The figure shows three views and two pictorial views of one solid part (mm, origin at its lowest corner). Answer the questions. Coordinates: 2 decimals unless noted, no trailing zeros. Loops run counter-clockwise (first coordinate to the right, second up) from the corner with the lowest first, then second, coordinate; pieces in that order, holes last. Notation, with made-up numbers: M 19,35 L 64,35 A34 ccw 64,72 Z; hole C 78.5,32 d1. An arc over 180 degrees is marked long. Return JSON: item names as keys, results as strings. Group by question number.
1. Section D-D (x = 28.5) is taken. Write down the section's boundary in (y, z).
2. Straight lines are drawn through the part: L1, parallel to Z at x = 3, y = 8; L2, parallel to Z at x = 12, y = 2.5; L3, parallel to X at y = 3.5, z = 6.5. For each, find the intervals that lie inside material, in ascending order. Write a range as from..to.
3. Section A-A (z = 15) is taken. Write down the section's boundary in (x, y), then the cut area to 3 significant figures.
4. Section B-B (x = 15) is taken. Write down the section's boundary in (y, z).
5. Given P1, Ø3.5, axis at x = 27, z = 3, coming from the +Y side, flat-ended and moving along its own axis, determine where the tip first touches the part or whether it passes through.
6. Section C-C (y = 1.25) is taken. Write down the section's boundary in (x, z), then the cut area to 3 significant figures.
7. The mould has two halves that part along Z. Classify the marked faces 1, 2 and 3: pulls with the +Z half, pulls with the -Z half, needs draft (parallel to the pull), parting line crosses it, or undercut.
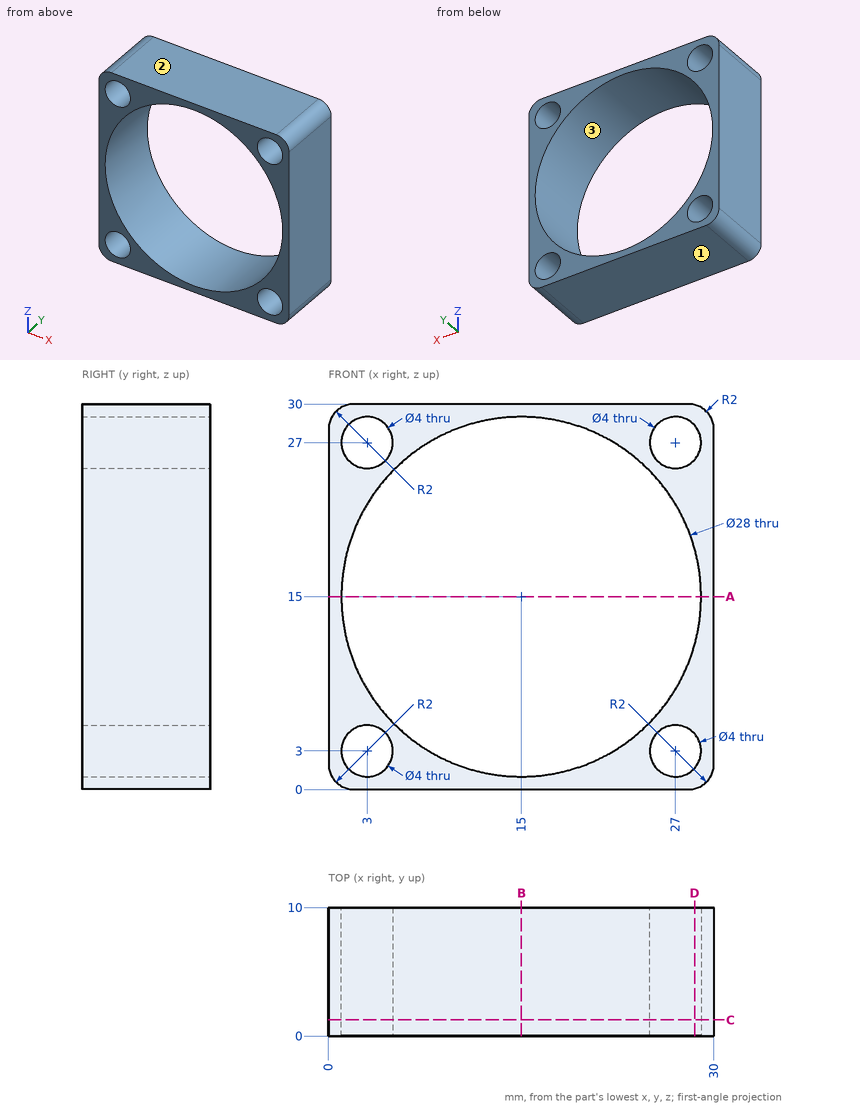
Worked out:
{
 "1": {"outline": "M 0,0.06 L 10,0.06 L 10,1.68 L 0,1.68 Z; M 0,4.32 L 10,4.32 L 10,11.29 L 0,11.29 Z; M 0,18.71 L 10,18.71 L 10,25.68 L 0,25.68 Z; M 0,28.32 L 10,28.32 L 10,29.94 L 0,29.94 Z"},
 "2": {"L1": "0..1, 5..7.79, 22.21..25, 29..30", "L2": "0..1.33, 28.67..30", "L3": "0..3.88, 26.12..30"},
 "3": {"outline": "M 0,0 L 1,0 L 1,10 L 0,10 Z; M 29,0 L 30,0 L 30,10 L 29,10 Z", "area": "20.0 mm^2"},
 "4": {"outline": "M 0,0 L 10,0 L 10,1 L 0,1 Z; M 0,29 L 10,29 L 10,30 L 0,30 Z"},
 "5": {"P1": "through"},
 "6": {"outline": "M 0,2 A2 ccw 2,0 L 28,0 A2 ccw 30,2 L 30,28 A2 ccw 28,30 L 2,30 A2 ccw 0,28 Z; hole C 3,3 d4; hole C 15,15 d28; hole C 3,27 d4; hole C 27,3 d4; hole C 27,27 d4", "area": "231 mm^2"},
 "7": {"face 1": "pulls with the -Z half", "face 2": "pulls with the +Z half", "face 3": "undercut"}
}
